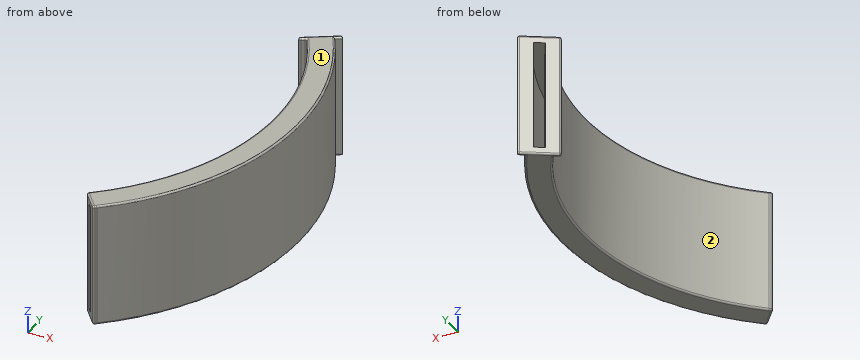
from build123d import *

# Parameters (mm, degrees)
SKETCH10_W          = 3.5
SKETCH10_H          = 17.5
SHELL1_T            = -1
SKETCH11_W          = 5.5
SKETCH11_H          = 17.5
SKETCH11_W_2        = 1.5
SKETCH11_H_2        = 15.5
BOSS_EXTRUDE1_DEPTH = 0.5
SKETCH12_W          = 15.5
SKETCH12_H          = 0.35
SKETCH12_W_2        = 1
SKETCH12_H_2        = 0.8
BOSS_EXTRUDE2_DEPTH = 0.5
FILLET1_R           = 0.25


with BuildPart() as part:
    # Sweep1: sweep along a path in Sketch7
    with BuildLine(Plane.XY) as sweep1_path:
        ThreePointArc((11.723892809, 0.886599981), (16.638600451, -22.580062041), (5.082270205, -43.586961119))
    # Sketch10 → Sweep1 (sweep)
    with BuildSketch(Plane(origin=(0, -17.481848747, 0), x_dir=(1, 0, 0), z_dir=(0, 1, 0))):
        with Locations((18.767181512, 0)):
            Rectangle(SKETCH10_W, SKETCH10_H)
    sweep(path=sweep1_path.line)

    # Shell1
    shell1_openings = [part.faces().sort_by_distance(p)[0] for p in [
        (6.227177499, -44.910474357, 0),
        (13.205526307, 1.817869101, 0),
    ]]
    offset(amount=SHELL1_T, openings=shell1_openings, kind=Kind.INTERSECTION)

    # Sketch11 → Boss-Extrude1 (add)
    with BuildSketch(Plane(origin=(2.920606872, -4.646636383, 0), x_dir=(0.8466477136319881, 0.5321537832259836, 0), z_dir=(-0.5321537832259836, 0.8466477136319881, 0))):
        with Locations((12.147814575, 0)):
            Rectangle(SKETCH11_W, SKETCH11_H)
        with Locations((12.147814575, 0)):
            Rectangle(SKETCH11_W_2, SKETCH11_H_2, mode=Mode.SUBTRACT)
    extrude(amount=BOSS_EXTRUDE1_DEPTH)

    # Sketch12 → Boss-Extrude2 (add)
    with BuildSketch(Plane(origin=(-18.659517469, -16.141446142, 0), x_dir=(0, 0, 1), z_dir=(-0.7562932785342891, -0.654232739049229, 0))):
        Polygon((-7.75, -38.439513283), (-8.75, -38.439513283), (-8.75, -39.789513283), (8.75, -39.789513283), (8.75, -38.439513283), (7.75, -38.439513283), (7.75, -38.789513283), (-7.75, -38.789513283), align=None)
        with Locations((0, -38.614513283)):
            Rectangle(SKETCH12_W, SKETCH12_H)
        Polygon((8.75, -36.289513283), (-8.75, -36.289513283), (-8.75, -37.639513283), (-7.75, -37.639513283), (-7.75, -37.289513283), (7.75, -37.289513283), (7.75, -37.639513283), (8.75, -37.639513283), align=None)
        with Locations((0, -37.464513283)):
            Rectangle(SKETCH12_W, SKETCH12_H)
        with Locations((8.25, -38.039513283)):
            Rectangle(SKETCH12_W_2, SKETCH12_H_2)
        with Locations((-8.25, -38.039513283)):
            Rectangle(SKETCH12_W_2, SKETCH12_H_2)
    extrude(amount=BOSS_EXTRUDE2_DEPTH)

    # Fillet1
    fillet1_edges = [part.edges().sort_by_distance(p)[0] for p in [
        (16.638600451, -22.580062041, -8.75),
        (16.638600451, -22.580062041, 8.75),
        (20.100212795, -23.097014635, 8.75),
        (20.100212795, -23.097014635, -8.75),
        (15.267730628, 3.704615862, 0),
        (12.939449416, 2.241192958, -8.75),
        (10.611168203, 0.777770054, 0),
        (12.939449416, 2.241192958, 8.75),
        (15.400769074, 3.492953934, 8.75),
        (15.110483663, 3.015215114, -8.75),
        (11.300568952, 0.620523089, -8.75),
        (15.400769074, 3.492953934, -8.75),
        (10.877245095, 0.354446198, 0),
        (10.744206649, 0.566108126, -8.75),
        (11.300568952, 0.620523089, 8.75),
        (15.110483663, 3.015215114, 8.75),
        (10.744206649, 0.566108126, 8.75),
        (11.723892809, 0.886599981, 0),
        (4.893196886, -43.750519304, 8.75),
        (4.893196886, -43.750519304, -8.75),
        (7.183011472, -46.397545779, -8.75),
        (7.183011472, -46.397545779, 8.75),
        (4.704123566, -43.914077489, 0),
        (5.849030859, -45.237590726, -8.75),
        (6.993938153, -46.561103964, 0),
        (5.849030859, -45.237590726, 8.75),
    ]]
    fillet(fillet1_edges, radius=FILLET1_R - 0.0001)  # a hair under: the kernel refuses the full size


solid = part.part
Geometry check sheet. Reference: the model listing, model coordinates, mm. Face numbers are marked on the shaded views. Coordinates: 2 decimals unless noted, no trailing zeros. One line per item, written item: value.
(1) Thickness scan on probe 1 along Y at (x, z) = (11.25, 5); probe 2 along Y at (x, z) = (10.75, 6.5); probe 3 along X at (y, z) = (-5.5, -2.5). Record the ranges inside material, lowest first. Write a range as from..to.
Data:
probe 1: y = -42.36..-40.8, -38.34..-36.58, 0.59..1.18
probe 2: y = -42.92..-41.4, -39.01..-37.32, 0.56..0.84
probe 3: x = 14.87..15.94, 17.52..18.58
(2) Sectioned sample at B-B (x = 16.25). Count the separate pieces of the cut face and the enclosed holes in it, and give its area (3 significant figures).
Data:
separate pieces: 2
enclosed holes: 2
area: 230 mm^2
(3) Release check for a two-part mould opening along Y. For the marked faces 1 and 2 record: +Y half, -Y half, draft (parallel to the pull), parting line (faces both ways), or undercut.
Data:
face 1: draft
face 2: undercut
(4) Depth check by flat-ended pin: pin 1 Ø4 at (x, z) = (17.5, 3) entering from -Y; pin 2 Ø5 at (x, y) = (18.5, -31.5) entering from +Z; pin 3 Ø5 at (y, z) = (-40, -0.5) entering from -X; pin 4 Ø6 at (x, z) = (11.5, -2.5) entering from +Y. Enter the tip coordinate at first touch or a pass-through.
Data:
pin 1: stops at y = -36.36
pin 2: stops at z = 8.75
pin 3: stops at x = 6.28
pin 4: stops at y = 3.22
